from build123d import *

# Parameters (mm, degrees)
SKETCH_1_R          = 9.55
SKETCH_1_R_2        = 3.6
EXTRUDE_1_DEPTH     = 8.4
SKETCH_2_R          = 4.3
CUT_EXTRUDE_1_DEPTH = 0.8


with BuildPart() as part:
    # 스케치1 → 보스-돌출1 (new body, symmetric)
    with BuildSketch(Plane.XY):
        Circle(SKETCH_1_R)
        Circle(SKETCH_1_R_2, mode=Mode.SUBTRACT)
    extrude(amount=EXTRUDE_1_DEPTH, both=True)

    # 스케치2 → 컷-돌출1 (cut)
    with BuildSketch(Plane.XY.offset(8.4)):
        Circle(SKETCH_2_R)
    cut_extrude_1 = extrude(amount=-CUT_EXTRUDE_1_DEPTH, mode=Mode.SUBTRACT)

    # 스케치3 → 컷-회전1 (revolve, cut)
    with BuildSketch(Plane(origin=(0, 0, 0), x_dir=(0, 0, -1), z_dir=(1, 0, 0))):
        Polygon((-8.4, 9.55), (-5.9, 9.55), (-7.15, 8.25), align=None)
    cut_revolve_1 = revolve(axis=Axis((0, 0, 0), (0, 0, 1)), mode=Mode.SUBTRACT)

    # 대칭 복사1: 컷-돌출1, 컷-회전1 across plane
    add(cut_extrude_1.mirror(Plane.XY), mode=Mode.SUBTRACT)
    add(cut_revolve_1.mirror(Plane.XY), mode=Mode.SUBTRACT)


solid = part.part
For this review, take the finished solid that the model builds, in its own axes (mm). A direction names the side the tool comes from. Round coordinates to 2 decimals unless told otherwise and drop trailing zeros. Order: outer loops, then holes, each group sorted by start corner. A loop starts at its lowest first (then second) coordinate and runs counter-clockwise, first axis right, second up. Notation, with made-up numbers: M -18.75,57 L 39.25,57 A21 ccw 39.25,62 Z; hole C 60,53 d11. An arc over 180 degrees is marked long. Write each question's results on one line, items separated by ' | '. Start each with the question number.
1. To check wall thickness, follow L1, parallel to Y at x = 0, z = -3.25; L2, parallel to Z at x = -7.5, y = 4; L3, parallel to Y at x = 1, z = 1.5. State the ranges of each line that lie inside material, in increasing order. Write a range as [from, to].
2. Draft analysis for pull direction X (two halves, no side actions). For faces 3 (the face through (4, -2, 8.4)), 4 (the face through (-4.296, 0.189, 8.006)), 5 (the face through (8.82, -3.66, 0.08)), state which applies: pulls with the +X half, pulls with the -X half, needs draft (parallel to the pull), parting line crosses it, or undercut.
3. Add section A-A (y = 0). State the section outline as (x, z) points, then the cut area to 3 significant figures.
4. Clearance check with flat-ended pins moving along their axes: pin 1 Ø2 at (x, z) = (-4.5, -4) entering from +Y; pin 2 Ø7 at (x, y) = (-0.5, 0.5) entering from -Z; pin 3 Ø6 at (x, y) = (0, 0) entering from +Z; pin 4 Ø3 at (x, y) = (-0.5, -2.5) entering from +Z. State where each tip first meets the part, or that it passes through.
5. Tool access review of faces 1 (the face through (-4.296, 0.189, -8.006)), 2 (the face through (3.434, 1.081, -0.106)): name each direction out of +Z, -Z, +X, -X, +Y, -Y from which nothing blocks a thin tool from reaching the whole face with its end or side.
6. Add section B-B (z = 3.5). State the section outline as (x, y) points.
Output values:
1) L1: [-9.55, -3.6], [3.6, 9.55] | L2: [-8.4, -7.39], [-6.91, 6.91], [7.39, 8.4] | L3: [-9.5, -3.46], [3.46, 9.5]
2) face 3: needs draft | face 4: undercut | face 5: parting line crosses it
3) outline: M -9.55,-8.4 L -4.3,-8.4 L -4.3,-7.6 L -3.6,-7.6 L -3.6,7.6 L -4.3,7.6 L -4.3,8.4 L -9.55,8.4 L -8.25,7.15 L -9.55,5.9 L -9.55,-5.9 L -8.25,-7.15 Z; M 3.6,-7.6 L 4.3,-7.6 L 4.3,-8.4 L 9.55,-8.4 L 8.25,-7.15 L 9.55,-5.9 L 9.55,5.9 L 8.25,7.15 L 9.55,8.4 L 4.3,8.4 L 4.3,7.6 L 3.6,7.6 Z | area: 191 mm^2
4) pin 1: y = 8.89 | pin 2: z = -7.6 | pin 3: through | pin 4: z = 7.6
5) face 1: -Z | face 2: +Z, -Z
6) outline: C 0,0 d19.1; hole C 0,0 d7.2
